```python
from build123d import *

# Parameters (mm, degrees)
ESQUISSE1_R        = 1.5
BOSS_EXTRU_1_DEPTH = 2.5


with BuildPart() as part:
    # Esquisse1 → Boss.-Extru.1 (new body)
    with BuildSketch(Plane(origin=(0, 0, 0), x_dir=(0, 0, -1), z_dir=(1, 0, 0))):
        with BuildLine():
            Line((-9.317485624, -34.773329746), (-9.317485624, -45.403821003))
            ThreePointArc((-9.317485624, -45.403821003), (-14.870482968, -43.89978629), (-20.194379814, -41.719414233))
            ThreePointArc((-20.194379814, -41.719414233), (-21.229656255, -38.966646831), (-22.782160988, -36.468796809))
            ThreePointArc((-22.782160988, -36.468796809), (0, 43), (22.782160988, -36.468796809))
            ThreePointArc((22.782160988, -36.468796809), (21.229656255, -38.966646831), (20.194379814, -41.719414233))
            ThreePointArc((20.194379814, -41.719414233), (14.870482968, -43.89978629), (9.317485624, -45.403821003))
            Line((9.317485624, -45.403821003), (9.317485624, -34.773329746))
            ThreePointArc((9.317485624, -34.773329746), (0, 36), (-9.317485624, -34.773329746))
        make_face()
        with Locations((-15.826054686, -39.441057647)):
            Circle(ESQUISSE1_R, mode=Mode.SUBTRACT)
        with Locations(Location((15.826054686, -39.441057647, 0), (0, 0, 180))):
            Circle(ESQUISSE1_R, mode=Mode.SUBTRACT)
    extrude(amount=BOSS_EXTRU_1_DEPTH)


solid = part.part
```
Could you check a few things on this model? Use its own coordinates, in mm. A direction names the side the tool comes from. Coordinates: 2 decimals unless noted, no trailing zeros. Order: outer loops, then holes, each group sorted by start corner. A loop starts at its lowest first (then second) coordinate and runs counter-clockwise, first axis right, second up. Notation, with made-up numbers: M -35.75,26 L -11.75,26 A27 cw -11.75,49 Z; hole C 72.25,45 d7. An arc over 180 degrees is marked long. Use a Markdown table: item, result. Add a question column.
Q1. We'd pull the mould along Z, two halves only. Please class faces 1 (the flat face through (0, -17, -32)), 2 (the cylindrical face through (1.232, -43.926, 14.794)), 3 (the cylindrical face through (1.23, -40.93, -16.02)): pulls with the +Z half, pulls with the -Z half, needs draft (parallel to the pull), parting line crosses it, or undercut.
Q2. Which directions (+Z, -Z, +X, -X, +Y, -Y) give clear straight access to the entire face, cutting with the end or side of a thin tool? Please do faces 4 (the flat face through (1, -40, 9.317)), 5 (the cylindrical face through (1.232, -40.905, 16.151)).
Q3. I want a section at C-C on x = 1.8. List the corners of the cut face in (y, z) for me.
Q4. If I drill on L1, parallel to Z at x = 1.8, y = -8; L2, parallel to Z at x = 1.7, y = 0; L3, parallel to Y at x = 0.9, z = -11, over which ranges is the centre line in solid material (lowest first)?
Q5. I want a section at D-D on z = 0. List the corners of the cut face in (x, y) for me, then the cut area to 3 significant figures.
Q6. I'm going to push flat-ended pins straight in: pin 1 (1.5 mm diameter, centred on x = 1, y = 16.5, fed in from -Z); pin 2 (1.5 mm diameter, centred on x = 2, z = 25.5, fed in from -Y); pin 3 (1.5 mm diameter, centred on x = 2, y = 17, fed in from +Z). Where does each tip first touch, or does it pass through?
Q7. I want a section at B-B on y = 0. List the corners of the cut face in (x, z) for me.
Q8. I want a section at A-A on z = -13. List the corners of the cut face in (x, y) for me.
Checked values:
| question | item | result |
|---|---|---|
| 1 | face 1 | needs draft |
| 1 | face 2 | pulls with the +Z half |
| 1 | face 3 | undercut |
| 2 | face 4 | +X, -X, -Y |
| 2 | face 5 | +X, -X |
| 3 | outline | M -45.4,-9.32 A46.35 ccw -41.72,-20.19 A15 cw -36.47,-22.78 A43 ccw long -36.47,22.78 A15 cw -41.72,20.19 A46.35 ccw -45.4,9.32 L -34.77,9.32 A36 cw long -34.77,-9.32 Z; hole C -39.44,-15.83 d3; hole C -39.44,15.83 d3 |
| 4 | L1 | -42.25 to -35.1, 35.1 to 42.25 |
| 4 | L2 | -43 to -36, 36 to 43 |
| 4 | L3 | -45.03 to -34.28, 34.28 to 41.57 |
| 5 | outline | M 0,36 L 2.5,36 L 2.5,43 L 0,43 Z |
| 5 | area | 17.5 mm² |
| 6 | pin 1 | z = -40.01 |
| 6 | pin 2 | y = -35.16 |
| 6 | pin 3 | z = 39.81 |
| 7 | outline | M 0,-43 L 2.5,-43 L 2.5,-36 L 0,-36 Z; M 0,36 L 2.5,36 L 2.5,43 L 0,43 Z |
| 8 | outline | M 0,-44.49 L 2.5,-44.49 L 2.5,-33.57 L 0,-33.57 Z; M 0,33.57 L 2.5,33.57 L 2.5,40.99 L 0,40.99 Z |
